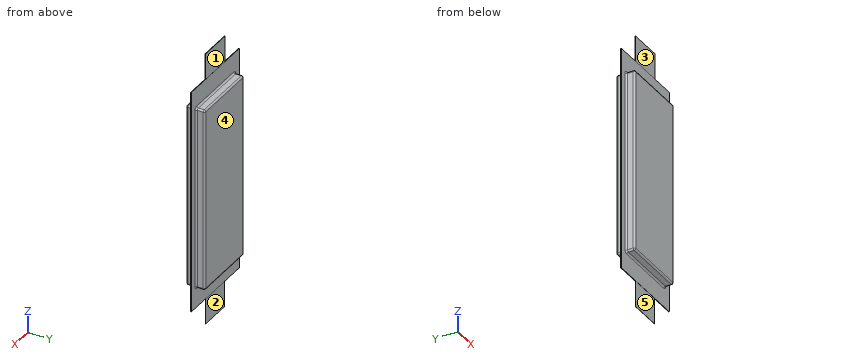
```python
from build123d import *

# Parameters (mm, degrees)
SKETCH1_W                = 40.6
SKETCH1_H                = 113
BOSS_EXTRUDE2_DEPTH      = 11.4
SKETCH3_W                = 4.7
SKETCH3_H                = 0.01
BOSS_EXTRUDE3_DEPTH      = 1
BOSS_EXTRUDE4_DEPTH      = 0.185
BOSS_EXTRUDE4_DEPTH_BACK = 0.185
SKETCH4_W                = 50
SKETCH4_H                = 138.2
BOSS_EXTRUDE5_DEPTH      = 16
BOSS_EXTRUDE6_DEPTH      = 16
FILLET1_R                = 1


with BuildPart() as part:
    # Sketch1 → Boss-Extrude2 (new body)
    with BuildSketch(Plane(origin=(0, 0, 0), x_dir=(1, 0, 0), z_dir=(0, 1, 0))):
        with Locations((20.3, 56.5)):
            Rectangle(SKETCH1_W, SKETCH1_H)
    extrude(amount=BOSS_EXTRUDE2_DEPTH)



with BuildPart() as body_2:
    # Sketch3 → Boss-Extrude3 (new body)
    with BuildSketch(Plane.XY):
        with Locations((-2.35, 5.695)):
            Rectangle(SKETCH3_W, SKETCH3_H)
    extrude(amount=BOSS_EXTRUDE3_DEPTH)


with BuildPart() as part_1:
    add(part.part)

    add(body_2.part)  # Boss-Extrude4 merges body 2
    # Sketch4 → Boss-Extrude4 (add, two sides: drawn at the far end of the back side and taken through both)
    with BuildSketch(Plane(origin=(0, 5.7, 0), x_dir=(1, 0, 0), z_dir=(0, 1, 0)).offset(-BOSS_EXTRUDE4_DEPTH_BACK)):
        with Locations((20.3, 56.5)):
            Rectangle(SKETCH4_W, SKETCH4_H)
    extrude(amount=BOSS_EXTRUDE4_DEPTH + BOSS_EXTRUDE4_DEPTH_BACK)

    # Sketch5 → Boss-Extrude5 (add)
    with BuildSketch(Plane.XY.offset(12.6)):
        Polygon((30.4, 5.85), (20.3, 5.85), (10.2, 5.85), (10.2, 5.549950483), (30.4, 5.549950483), align=None)
    extrude(amount=BOSS_EXTRUDE5_DEPTH)

    # Sketch6 → Boss-Extrude6 (add)
    with BuildSketch(Plane(origin=(0, 0, -125.6), x_dir=(-1, 0, 0), z_dir=(0, 0, -1))):
        Polygon((-20.3, 5.765), (-10.35, 5.765), (-10.35, 5.635), (-30.25, 5.635), (-30.25, 5.765), align=None)
    extrude(amount=BOSS_EXTRUDE6_DEPTH)

    # Fillet1
    fillet1_edges = [part_1.edges().sort_by_distance(p)[0] for p in [
        (40.6, 11.4, -56.5),
        (20.3, 11.4, -113),
        (0, 2.7575, -113),
        (40.6, 2.7575, -113),
        (20.3, 5.885, -113),
        (20.3, 5.515, -113),
        (40.6, 2.7575, 0),
        (0, 2.7575, 0),
        (20.3, 5.885, 0),
        (0, 5.885, -56.5),
        (40.6, 5.885, -56.5),
        (20.3, 5.515, 0),
        (0, 5.515, -56.5),
        (40.6, 5.515, -56.5),
        (0, 11.4, -56.5),
        (20.3, 0, -113),
        (40.6, 0, -56.5),
        (20.3, 0, 0),
        (0, 0, -56.5),
        (20.3, 11.4, 0),
        (0, 8.6425, -113),
        (40.6, 8.6425, -113),
        (40.6, 8.6425, 0),
        (0, 8.6425, 0),
    ]]
    fillet(fillet1_edges, radius=FILLET1_R)


solid = part_1.part
```
Build history of the part. All positions in model axes, mm. Face numbers are marked on the shaded views. A direction names the side the tool comes from. Coordinates: 2 decimals unless noted, no trailing zeros. Order: outer loops, then holes, each group sorted by start corner. A loop starts at its lowest first (then second) coordinate and runs counter-clockwise, first axis right, second up.
Item 1: Saw through at D-D on x = 4.5. List the corners of the cut face in (y, z) (3 decimals).
Filled in:
outline: (0, -112) arc R1 ccw to (1, -113) - (4.515, -113) arc R1 cw to (5.515, -114) - (5.515, -125.6) - (5.885, -125.6) - (5.885, -114) arc R1 cw to (6.885, -113) - (10.4, -113) arc R1 ccw to (11.4, -112) - (11.4, -1) arc R1 ccw to (10.4, 0) - (6.885, 0) arc R1 cw to (5.885, 1) - (5.885, 12.6) - (5.515, 12.6) - (5.515, 1) arc R1 cw to (4.515, 0) - (1, 0) arc R1 ccw to (0, -1) - close
Item 2: Drop flat-ended pins along their axis: pin 1 Ø3 at (y, z) = (8, -65.5) entering from -X; pin 2 Ø1.8 at (x, y) = (23, 8.5) entering from -Z; pin 3 Ø4 at (x, z) = (30, -65) entering from -Y; pin 4 Ø13 at (x, z) = (16, -137.5) entering from +Y (3 decimals). Give the stop position or say it passes through.
Filled in:
pin 1: stops at x = -0.08
pin 2: stops at z = -113
pin 3: stops at y = 0
pin 4: stops at y = 5.765
Item 3: Drill centre lines: L1, parallel to X at y = 3.25, z = -88; L2, parallel to Z at x = 25.5, y = 8.25; L3, parallel to Y at x = 42, z = -1.5 (3 decimals). Where is each one in solid material? Low to high.
Filled in:
L1: x = 0 to 40.6
L2: z = -113 to 0
L3: y = 5.515 to 5.885
Item 4: Tool access for the marked faces 1, 2, 3, 4 and 5: list every direction of +Z, -Z, +X, -X, +Y, -Y with a clear straight run to the whole face (end or side of a thin tool).
Filled in:
face 1: +Z, +X, -X, +Y
face 2: -Z, +X, -X, +Y
face 3: +Z, +X, -X, -Y
face 4: +Z, -Z, +X, -X, +Y
face 5: -Z, +X, -X, -Y
Item 5: Saw through at C-C on y = 2.5. List the corners of the cut face in (x, z), then the cut area to 3 significant figures.
Filled in:
outline: (0, -112) arc R1 ccw to (1, -113) - (39.6, -113) arc R1 ccw to (40.6, -112) - (40.6, -1) arc R1 ccw to (39.6, 0) - (1, 0) arc R1 ccw to (0, -1) - close
area: 4,590 mm2
Item 6: Saw through at A-A on x = 22.5. List the corners of the cut face in (y, z) (3 decimals).
Filled in:
outline: (0, -112) arc R1 ccw to (1, -113) - (4.515, -113) arc R1 cw to (5.515, -114) - (5.515, -125.6) - (5.635, -125.6) - (5.635, -141.6) - (5.765, -141.6) - (5.765, -125.6) - (5.885, -125.6) - (5.885, -114) arc R1 cw to (6.885, -113) - (10.4, -113) arc R1 ccw to (11.4, -112) - (11.4, -1) arc R1 ccw to (10.4, 0) - (6.885, 0) arc R1 cw to (5.885, 1) - (5.885, 12.6) - (5.85, 12.6) - (5.85, 28.6) - (5.55, 28.6) - (5.55, 12.6) - (5.515, 12.6) - (5.515, 1) arc R1 cw to (4.515, 0) - (1, 0) arc R1 ccw to (0, -1) - close
Item 7: Saw through at B-B on z = -5. List the corners of the cut face in (x, y) (3 decimals), then the cut area to 3 significant figures.
Filled in:
outline: (-4.7, 5.515) - (-1, 5.515) arc R1 cw to (0, 4.515) - (0, 1) arc R1 ccw to (1, 0) - (39.6, 0) arc R1 ccw to (40.6, 1) - (40.6, 4.515) arc R1 cw to (41.6, 5.515) - (45.3, 5.515) - (45.3, 5.885) - (41.6, 5.885) arc R1 cw to (40.6, 6.885) - (40.6, 10.4) arc R1 ccw to (39.6, 11.4) - (1, 11.4) arc R1 ccw to (0, 10.4) - (0, 6.885) arc R1 cw to (-1, 5.885) - (-4.7, 5.885) - close
area: 466 mm2
